Model file for the job. Use its own axes, mm. A direction names the side the tool comes from. Coordinates: 2 decimals unless noted, no trailing zeros. Order: outer loops, then holes, each group sorted by start corner. A loop starts at its lowest first (then second) coordinate and runs counter-clockwise, first axis right, second up. Notation, with made-up numbers: (22.5, 24) -> (74.5, 24) arc R13 ccw to (74.5, 48) -> close; hole circle Ø2 at (-0.75, 76). An arc over 180 degrees is marked (long way). Return JSON: item names as keys, results as strings. Group by question number.
1) Cut at A-A (z = -64). Write the cut outline in (x, y).
2) Flat gauge pins, fed straight in: pin 1 (12 mm diameter, centred on y = 23, z = -54, fed in from -X); pin 2 (1.5 mm diameter, centred on y = -38, z = -47.5, fed in from +X); pin 3 (3 mm diameter, centred on y = 18, z = -22, fed in from -X); pin 4 (4 mm diameter, centred on y = -0.5, z = -50, fed in from +X). Where does each tip first touch, or does it go through?
3) Pull direction X, two halves, no side cores. Call faces 1 (the flat face through (6, -30, -30)), 2 (the cylindrical face through (45.783, -14.418, -45.63)), 3 (the flat face through (-0.2, 42.4, -90)): +X half, -X half, draft (parallel to the pull), parting line (faces both ways), or undercut.
4) Probe line 1 (Y direction, x = 0, z = -76); line 2 (Y direction, x = 0, z = -6); line 3 (Z direction, x = -21.5, y = -32). List the from-to ranges inside material, lowest first.
5) Which spindle directions (+Z, -Z, +X, -X, +Y, -Y) get a long thin tool onto all of the face, cutting with end or side? Do faces 4 (the flat face through (-18, 21, -22)), 5 (the flat face through (-25, 28, 0)), 6 (the cylindrical face through (9.051, -40.757, -70.138)), 7 (the flat face through (-25, -11, -27)). Say none if no direction does.
6) Cut at B-B (z = -23.5). Write the cut outline in (x, y), and give its area (3 significant figures).
from build123d import *

# Parameters (mm, degrees)
SKETCH_2_R          = 36.5
CUT_EXTRUDE_1_DEPTH = 2
SKETCH_3_R          = 41.75
CUT_EXTRUDE_2_DEPTH = 2.3
FILLET_1_R          = 0.3
CHAMFER_2_SIZE      = 2


with BuildPart() as part:
    # Sketch 1 → Revolve 1 (revolve)
    with BuildSketch(Plane(origin=(0, 0, 0), x_dir=(0, 0, -1), z_dir=(1, 0, 0)), mode=Mode.PRIVATE) as revolve_1_sk:
        Polygon((0, 48), (90, 48), (90, 40), (30, 40), (30, 30), (27, 30), (27, 27), (22, 27), (22, 35), (0, 35), align=None)
    revolve(revolve_1_sk.sketch.rotate(Axis((0, 0, 0), (0, 0, -1)), 90), axis=Axis((0, 0, 0), (0, 0, -1)))

    # Sketch 2 → Cut-Extrude 1 (cut)
    with BuildSketch(Plane.XY.offset(-14)):
        Circle(SKETCH_2_R)
    extrude(amount=CUT_EXTRUDE_1_DEPTH, mode=Mode.SUBTRACT)

    # Sketch 3 → Cut-Extrude 2 (cut)
    with BuildSketch(Plane(origin=(0, 0, -69), x_dir=(-1, 0, 0), z_dir=(0, 0, -1))):
        Circle(SKETCH_3_R)
    extrude(amount=CUT_EXTRUDE_2_DEPTH, mode=Mode.SUBTRACT)

    # Fillet 1
    fillet_1_edges = [part.edges().sort_by_distance(p)[0] for p in [
        (-36.5, 0, -12),
        (-36.5, 0, -14),
        (41.75, 0, -71.3),
        (41.75, 0, -69),
    ]]
    fillet(fillet_1_edges, radius=FILLET_1_R)

    # Chamfer 2
    chamfer_2_edges = [part.edges().sort_by_distance(p)[0] for p in [
        (-40, 0, -90),
        (-35, 0, 0),
    ]]
    chamfer(chamfer_2_edges, length=CHAMFER_2_SIZE)


solid = part.part
Answers below:
{
 "1": {"outline": "circle Ø96 at (0, 0); hole circle Ø80 at (0, 0)"},
 "2": {"pin 1": "stops at x = -44.89", "pin 2": "stops at x = 30.27", "pin 3": "stops at x = -45.07", "pin 4": "stops at x = 48"},
 "3": {"face 1": "undercut", "face 2": "parting line", "face 3": "draft"},
 "4": {"line 1": "y = -48 to -40, 40 to 48", "line 2": "y = -48 to -35, 35 to 48", "line 3": "z = -30 to 0"},
 "5": {"face 4": "+Z", "face 5": "+Z, +X, -X, +Y, -Y", "face 6": "none", "face 7": "-Z"},
 "6": {"outline": "circle Ø96 at (0, 0); hole circle Ø54 at (0, 0)", "area": "4,950 mm^2"}
}
